Source: CAD feature listing. Evaluate the final solid. Frame: model axes, mm. Round coordinates to 2 decimals unless told otherwise and drop trailing zeros. Write each loop counter-clockwise with the first axis right and the second up, starting at its lowest first coordinate (ties: lowest second). Pieces come first, ordered by that corner, then holes. Notation, with made-up numbers: (-8, 75) -> (3, 75) arc R13 ccw to (3, 89) -> close; hole circle Ø1 at (78.5, 65.25). An arc over 180 degrees is marked (long way). Put each result on its own line as item: value.
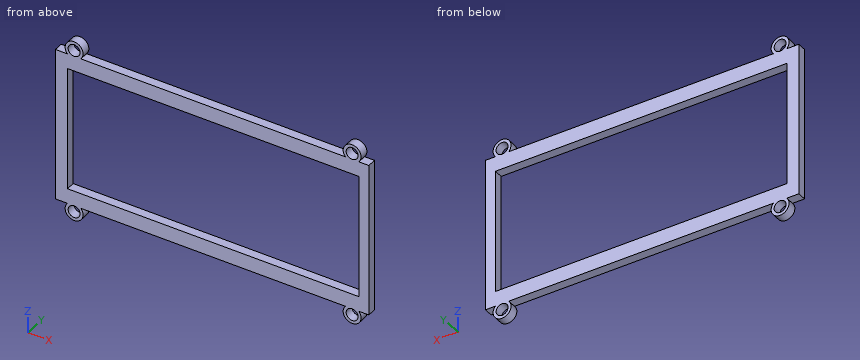
Autodesk Inventor part; units mm, degrees
ref_plane "YZ Plane" through (0, 0, 0) normal (1, 0, 0) x (0, 1, 0)
ref_plane "XZ Plane" through (0, 0, 0) normal (0, 1, 0) x (-1, 0, 0)
ref_plane "XY Plane" through (0, 0, 0) normal (0, 0, 1) x (1, 0, 0)
sketch "Sketch1" plane through (0, 0, 0) normal (0, 1, 0) x (-1, 0, 0)
  spline S0 degree 3 poles (-9.8463, -11.5333) (-9.7942, -11.6131) (-9.7348, -11.6874) (-9.6692, -11.7553) (-9.4724, -11.9589) (-9.2192, -12.1042) (-8.936, -12.1641) (-8.8416, -12.1841) (-8.7439, -12.1946) (-8.6437, -12.1946) (-8.5436, -12.1946) (-8.4459, -12.1841) (-8.3515, -12.1641) (-8.0682, -12.1042) (-7.8151, -11.9589) (-7.6183, -11.7553) (-7.5527, -11.6874) (-7.4933, -11.6131) (-7.4412, -11.5333) (-7.337, -11.3737) (-7.2616, -11.1922) (-7.223, -10.9969) (-7.2037, -10.8993) (-7.1935, -10.7982) (-7.1935, -10.6946) (-7.1935, -9.8662) (-7.8428, -9.1946) (-8.6437, -9.1946) (-9.4447, -9.1946) (-10.094, -9.8662) (-10.094, -10.6946) (-10.094, -10.7982) (-10.0838, -10.8993) (-10.0645, -10.9969) (-10.0259, -11.1922) (-9.9505, -11.3737) (-9.8463, -11.5333) knots 0 0 0 0 1 1 1 2 2 2 3 3 3 4 4 4 5 5 5 6 6 6 7 7 7 8 8 8 9 9 9 10 10 10 11 11 11 12 12 12 12
  line L0 (-9.8463, -11.5333) -> (-9.7942, -11.6131) construction
  line L1 (-9.7942, -11.6131) -> (-9.7348, -11.6874) construction
  line L2 (-9.7348, -11.6874) -> (-9.6692, -11.7553) construction
  line L3 (-9.6692, -11.7553) -> (-9.4724, -11.9589) construction
  line L4 (-9.4724, -11.9589) -> (-9.2192, -12.1042) construction
  line L5 (-9.2192, -12.1042) -> (-8.936, -12.1641) construction
  line L6 (-8.936, -12.1641) -> (-8.8416, -12.1841) construction
  line L7 (-8.8416, -12.1841) -> (-8.7439, -12.1946) construction
  line L8 (-8.7439, -12.1946) -> (-8.6437, -12.1946) construction
  line L9 (-8.6437, -12.1946) -> (-8.5436, -12.1946) construction
  line L10 (-8.5436, -12.1946) -> (-8.4459, -12.1841) construction
  line L11 (-8.4459, -12.1841) -> (-8.3515, -12.1641) construction
  line L12 (-8.3515, -12.1641) -> (-8.0682, -12.1042) construction
  line L13 (-8.0682, -12.1042) -> (-7.8151, -11.9589) construction
  line L14 (-7.8151, -11.9589) -> (-7.6183, -11.7553) construction
  line L15 (-7.6183, -11.7553) -> (-7.5527, -11.6874) construction
  line L16 (-7.5527, -11.6874) -> (-7.4933, -11.6131) construction
  line L17 (-7.4933, -11.6131) -> (-7.4412, -11.5333) construction
  line L18 (-7.4412, -11.5333) -> (-7.337, -11.3737) construction
  line L19 (-7.337, -11.3737) -> (-7.2616, -11.1922) construction
  line L20 (-7.2616, -11.1922) -> (-7.223, -10.9969) construction
  line L21 (-7.223, -10.9969) -> (-7.2037, -10.8993) construction
  line L22 (-7.2037, -10.8993) -> (-7.1935, -10.7982) construction
  line L23 (-7.1935, -10.7982) -> (-7.1935, -10.6946) construction
  line L24 (-7.1935, -10.6946) -> (-7.1935, -9.8662) construction
  line L25 (-7.1935, -9.8662) -> (-7.8428, -9.1946) construction
  line L26 (-7.8428, -9.1946) -> (-8.6437, -9.1946) construction
  line L27 (-8.6437, -9.1946) -> (-9.4447, -9.1946) construction
  line L28 (-9.4447, -9.1946) -> (-10.094, -9.8662) construction
  line L29 (-10.094, -9.8662) -> (-10.094, -10.6946) construction
  line L30 (-10.094, -10.6946) -> (-10.094, -10.7982) construction
  line L31 (-10.094, -10.7982) -> (-10.0838, -10.8993) construction
  line L32 (-10.0838, -10.8993) -> (-10.0645, -10.9969) construction
  line L33 (-10.0645, -10.9969) -> (-10.0259, -11.1922) construction
  line L34 (-10.0259, -11.1922) -> (-9.9505, -11.3737) construction
  line L35 (-9.9505, -11.3737) -> (-9.8463, -11.5333) construction
  spline S1 degree 3 poles (83.1689, -11.5333) (83.221, -11.6131) (83.2803, -11.6874) (83.3459, -11.7553) (83.5428, -11.9589) (83.7959, -12.1042) (84.0791, -12.1641) (84.1735, -12.1841) (84.2713, -12.1946) (84.3714, -12.1946) (84.4715, -12.1946) (84.5693, -12.1841) (84.6637, -12.1641) (84.9469, -12.1042) (85.2001, -11.9589) (85.3969, -11.7553) (85.4625, -11.6874) (85.5218, -11.6131) (85.574, -11.5333) (85.6782, -11.3737) (85.7536, -11.1922) (85.7922, -10.9969) (85.8115, -10.8993) (85.8217, -10.7982) (85.8217, -10.6946) (85.8217, -9.8662) (85.1724, -9.1946) (84.3714, -9.1946) (83.5705, -9.1946) (82.9212, -9.8662) (82.9212, -10.6946) (82.9212, -10.7982) (82.9313, -10.8993) (82.9506, -10.9969) (82.9893, -11.1922) (83.0646, -11.3737) (83.1689, -11.5333) knots 0 0 0 0 1 1 1 2 2 2 3 3 3 4 4 4 5 5 5 6 6 6 7 7 7 8 8 8 9 9 9 10 10 10 11 11 11 12 12 12 12
  line L36 (83.1689, -11.5333) -> (83.221, -11.6131) construction
  line L37 (83.221, -11.6131) -> (83.2803, -11.6874) construction
  line L38 (83.2803, -11.6874) -> (83.3459, -11.7553) construction
  line L39 (83.3459, -11.7553) -> (83.5428, -11.9589) construction
  line L40 (83.5428, -11.9589) -> (83.7959, -12.1042) construction
  line L41 (83.7959, -12.1042) -> (84.0791, -12.1641) construction
  line L42 (84.0791, -12.1641) -> (84.1735, -12.1841) construction
  line L43 (84.1735, -12.1841) -> (84.2713, -12.1946) construction
  line L44 (84.2713, -12.1946) -> (84.3714, -12.1946) construction
  line L45 (84.3714, -12.1946) -> (84.4715, -12.1946) construction
  line L46 (84.4715, -12.1946) -> (84.5693, -12.1841) construction
  line L47 (84.5693, -12.1841) -> (84.6637, -12.1641) construction
  line L48 (84.6637, -12.1641) -> (84.9469, -12.1042) construction
  line L49 (84.9469, -12.1042) -> (85.2001, -11.9589) construction
  line L50 (85.2001, -11.9589) -> (85.3969, -11.7553) construction
  line L51 (85.3969, -11.7553) -> (85.4625, -11.6874) construction
  line L52 (85.4625, -11.6874) -> (85.5218, -11.6131) construction
  line L53 (85.5218, -11.6131) -> (85.574, -11.5333) construction
  line L54 (85.574, -11.5333) -> (85.6782, -11.3737) construction
  line L55 (85.6782, -11.3737) -> (85.7536, -11.1922) construction
  line L56 (85.7536, -11.1922) -> (85.7922, -10.9969) construction
  line L57 (85.7922, -10.9969) -> (85.8115, -10.8993) construction
  line L58 (85.8115, -10.8993) -> (85.8217, -10.7982) construction
  line L59 (85.8217, -10.7982) -> (85.8217, -10.6946) construction
  line L60 (85.8217, -10.6946) -> (85.8217, -9.8662) construction
  line L61 (85.8217, -9.8662) -> (85.1724, -9.1946) construction
  line L62 (85.1724, -9.1946) -> (84.3714, -9.1946) construction
  line L63 (84.3714, -9.1946) -> (83.5705, -9.1946) construction
  line L64 (83.5705, -9.1946) -> (82.9212, -9.8662) construction
  line L65 (82.9212, -9.8662) -> (82.9212, -10.6946) construction
  line L66 (82.9212, -10.6946) -> (82.9212, -10.7982) construction
  line L67 (82.9212, -10.7982) -> (82.9313, -10.8993) construction
  line L68 (82.9313, -10.8993) -> (82.9506, -10.9969) construction
  line L69 (82.9506, -10.9969) -> (82.9893, -11.1922) construction
  line L70 (82.9893, -11.1922) -> (83.0646, -11.3737) construction
  line L71 (83.0646, -11.3737) -> (83.1689, -11.5333) construction
  line L72 (-14.2577, -12.5451) -> (-14.2577, -64.0273)
  line L73 (-14.2577, -64.0273) -> (90.783, -64.0273)
  line L74 (90.783, -64.0273) -> (90.783, -12.5451)
  line L75 (90.783, -12.5451) -> (-14.2577, -12.5451)
  spline S2 degree 3 poles (-8.6437, -64.2555) (-9.4447, -64.2555) (-10.094, -64.9271) (-10.094, -65.7555) (-10.094, -66.5839) (-9.4447, -67.2555) (-8.6437, -67.2555) (-7.8428, -67.2555) (-7.1935, -66.5839) (-7.1935, -65.7555) (-7.1935, -64.9271) (-7.8428, -64.2555) (-8.6437, -64.2555) knots 0 0 0 0 1 1 1 2 2 2 3 3 3 4 4 4 4
  line L76 (-8.6437, -64.2555) -> (-9.4447, -64.2555) construction
  line L77 (-9.4447, -64.2555) -> (-10.094, -64.9271) construction
  line L78 (-10.094, -64.9271) -> (-10.094, -65.7555) construction
  line L79 (-10.094, -65.7555) -> (-10.094, -66.5839) construction
  line L80 (-10.094, -66.5839) -> (-9.4447, -67.2555) construction
  line L81 (-9.4447, -67.2555) -> (-8.6437, -67.2555) construction
  line L82 (-8.6437, -67.2555) -> (-7.8428, -67.2555) construction
  line L83 (-7.8428, -67.2555) -> (-7.1935, -66.5839) construction
  line L84 (-7.1935, -66.5839) -> (-7.1935, -65.7555) construction
  line L85 (-7.1935, -65.7555) -> (-7.1935, -64.9271) construction
  line L86 (-7.1935, -64.9271) -> (-7.8428, -64.2555) construction
  line L87 (-7.8428, -64.2555) -> (-8.6437, -64.2555) construction
  spline S3 degree 3 poles (84.4193, -64.2555) (83.6184, -64.2555) (82.9691, -64.9271) (82.9691, -65.7555) (82.9691, -66.5839) (83.6184, -67.2555) (84.4193, -67.2555) (85.2203, -67.2555) (85.8695, -66.5839) (85.8695, -65.7555) (85.8695, -64.9271) (85.2203, -64.2555) (84.4193, -64.2555) knots 0 0 0 0 1 1 1 2 2 2 3 3 3 4 4 4 4
  line L88 (84.4193, -64.2555) -> (83.6184, -64.2555) construction
  line L89 (83.6184, -64.2555) -> (82.9691, -64.9271) construction
  line L90 (82.9691, -64.9271) -> (82.9691, -65.7555) construction
  line L91 (82.9691, -65.7555) -> (82.9691, -66.5839) construction
  line L92 (82.9691, -66.5839) -> (83.6184, -67.2555) construction
  line L93 (83.6184, -67.2555) -> (84.4193, -67.2555) construction
  line L94 (84.4193, -67.2555) -> (85.2203, -67.2555) construction
  line L95 (85.2203, -67.2555) -> (85.8695, -66.5839) construction
  line L96 (85.8695, -66.5839) -> (85.8695, -65.7555) construction
  line L97 (85.8695, -65.7555) -> (85.8695, -64.9271) construction
  line L98 (85.8695, -64.9271) -> (85.2203, -64.2555) construction
  line L99 (85.2203, -64.2555) -> (84.4193, -64.2555) construction
  point P0 (0, 0)
sketch "Sketch2" plane through (0, 0, 0) normal (0, 1, 0) x (-1, 0, 0)
  circle A0 centre (84.4532, -10.6585) radius 2
  circle A1 centre (-8.5926, -10.6585) radius 2
  circle A2 centre (-8.5926, -65.7836) radius 2
  circle A3 centre (84.4532, -65.7836) radius 2
  circle A4 centre (-8.5926, -10.6585) radius 3
  circle A5 centre (-8.5926, -65.7836) radius 3
  circle A6 centre (84.4532, -65.7836) radius 3
  circle A7 centre (84.4532, -10.6585) radius 3
  line L0 (-14.1634, -12.6585) -> (90.7016, -12.6585)
  line L1 (90.7016, -12.6585) -> (90.7016, -17.6585)
  line L2 (90.7016, -17.6585) -> (-14.1634, -17.6585)
  line L3 (-14.1634, -17.6585) -> (-14.1634, -12.6585)
  line L4 (90.7016, -63.7836) -> (-14.1634, -63.7836)
  line L5 (-14.1634, -63.7836) -> (-14.1634, -58.7836)
  line L6 (-14.1634, -58.7836) -> (90.7016, -58.7836)
  line L7 (90.7016, -58.7836) -> (90.7016, -63.7836)
  line L8 (-14.1634, -12.6585) -> (-10.8287, -12.6585)
  line L9 (-10.8287, -12.6585) -> (-10.8287, -63.7836)
  line L10 (-10.8287, -63.7836) -> (-14.1634, -63.7836)
  line L11 (-14.1634, -63.7836) -> (-14.1634, -12.6585)
  line L12 (86.6893, -12.6585) -> (90.7016, -12.6585)
  line L13 (90.7016, -12.6585) -> (90.7016, -63.7836)
  line L14 (90.7016, -63.7836) -> (86.6893, -63.7836)
  line L15 (86.6893, -63.7836) -> (86.6893, -12.6585)
  point P0 (0, 0)
  dimension "d5" = 6
  dimension "d7" = 6
  dimension "d0" = 4
  dimension "d1" = 4
  dimension "d2" = 4
  dimension "d3" = 4
  dimension "d4" = 6
  dimension "d6" = 6
  dimension "d8" = 5
  dimension "d9" = 5
extrude "Extrusion1" add sketch "Sketch2" along normal blind 3 contours L0 A7 | L0 A7 | A7 L15 L2 L9 A4 L0 | L0 L1 L2 L15 | L0 A4 | A4 L0 | L2 L13 L6 L15 | L9 L2 L3 L0 | L9 L6 L11 L2 | L15 A6 L4 A5 L9 L6 | L6 L7 L4 L15 | L9 L4 L5 L6 | L4 A6 | A6 L4 | L4 A5 | A5 L4
properties part number "lcd-spacer-model"
Q1. Pin query (flat end, axial travel): pin 1 (1.5 mm diameter, centred on x = -88.5, y = 1.5, fed in from -Z); pin 2 (3 mm diameter, centred on x = -84.45, z = -10.66, fed in from -Y); pin 3 (0.9 mm diameter, centred on x = -47.5, y = 2, fed in from +Z). Return the tip coordinate at first contact, or that it passes through.
Ans:
pin 1: stops at z = -63.78
pin 2: passes through
pin 3: stops at z = -12.66
Q2. Material intervals for line 1 (X direction, y = 1.9, z = -25); line 2 (Z direction, x = -42, y = 1.3); line 3 (X direction, y = 1.85, z = -11), sorted ascending. Write a range as [from, to].
Ans:
line 1: x = [-90.7, -86.69], [10.83, 14.16]
line 2: z = [-63.78, -58.78], [-17.66, -12.66]
line 3: x = [-87.43, -86.42], [-82.48, -81.47], [5.61, 6.62], [10.56, 11.57]
Q3. Cut plane B-B on z = -24. Output: boundary loops of the cut face in (x, y), and give its area (3 significant figures).
Ans:
outline: (-90.7, 0) -> (-86.69, 0) -> (-86.69, 3) -> (-90.7, 3) -> close; (10.83, 0) -> (14.16, 0) -> (14.16, 3) -> (10.83, 3) -> close
area: 22.0 mm^2
Q4. Cut plane A-A on x = -50. Output: boundary loops of the cut face in (y, z), and give its area (3 significant figures).
Ans:
outline: (0, -63.78) -> (3, -63.78) -> (3, -58.78) -> (0, -58.78) -> close; (0, -17.66) -> (3, -17.66) -> (3, -12.66) -> (0, -12.66) -> close
area: 30.0 mm^2
Q5. Cut plane C-C on y = 1.4. Output: boundary loops of the cut face in (x, z).
Ans:
outline: (-90.7, -63.78) -> (-86.69, -63.78) arc R3 ccw (long way) to (-82.22, -63.78) -> (6.36, -63.78) arc R3 ccw (long way) to (10.83, -63.78) -> (14.16, -63.78) -> (14.16, -12.66) -> (10.83, -12.66) arc R3 ccw (long way) to (6.36, -12.66) -> (-82.22, -12.66) arc R3 ccw (long way) to (-86.69, -12.66) -> (-90.7, -12.66) -> close; hole (-86.69, -58.78) -> (10.83, -58.78) -> (10.83, -17.66) -> (-86.69, -17.66) -> close; hole circle Ø4 at (-84.45, -65.78); hole circle Ø4 at (-84.45, -10.66); hole circle Ø4 at (8.59, -65.78); hole circle Ø4 at (8.59, -10.66)
